```python
from build123d import *

# Parameters (mm, degrees)
SKETCH1_R           = 6.35
BOSS_EXTRUDE1_DEPTH = 38.1
SKETCH2_R           = 9.525
BOSS_EXTRUDE2_DEPTH = 12.7
CUT_EXTRUDE1_DEPTH  = 6.223


with BuildPart() as part:
    # Sketch1 → Boss-Extrude1 (new body)
    with BuildSketch(Plane(origin=(0, 0, 0), x_dir=(0, 0, -1), z_dir=(1, 0, 0))):
        Circle(SKETCH1_R)
    extrude(amount=-BOSS_EXTRUDE1_DEPTH)

    # Sketch2 → Boss-Extrude2 (add)
    with BuildSketch(Plane(origin=(0, 0, 0), x_dir=(0, 0, -1), z_dir=(1, 0, 0))):
        Circle(SKETCH2_R)
    extrude(amount=BOSS_EXTRUDE2_DEPTH)

    # Sketch3 → Cut-Extrude1 (cut)
    with BuildSketch(Plane(origin=(12.7, 0, 0), x_dir=(0, 0, -1), z_dir=(1, 0, 0))):
        Polygon((2.749630657, 4.7625), (-2.749630657, 4.7625), (-5.499261314, 0), (-2.749630657, -4.7625), (2.749630657, -4.7625), (5.499261314, 0), align=None)
    extrude(amount=-CUT_EXTRUDE1_DEPTH, mode=Mode.SUBTRACT)


solid = part.part
```
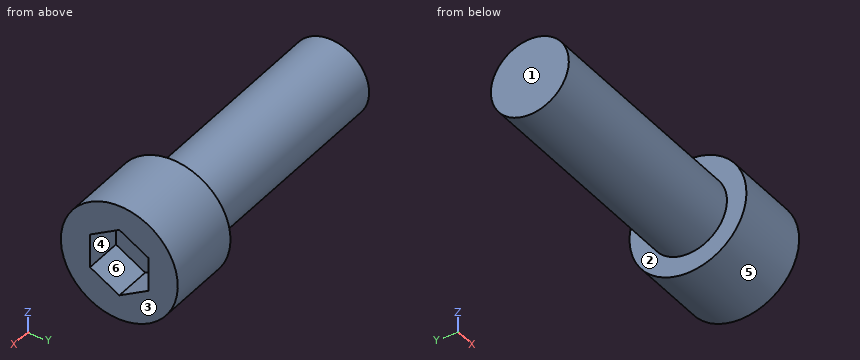
Design review of the part built by this model. Coordinates are the model's own, in mm. Face numbers are marked on the shaded views. A direction names the side the tool comes from. Give positions to 0.01 mm unless a question says otherwise; leave off trailing zeros. Loops run counter-clockwise (first coordinate to the right, second up) from the corner with the lowest first, then second, coordinate; pieces in that order, holes last. Notation, with made-up numbers: (53, 21.25) -> (105, 21.25) arc R18 cw to (105, 36.25) -> close; hole circle Ø11 at (78.25, -21). An arc over 180 degrees is marked (long way). One line per item, written item: value.
Q1. Draft analysis for pull direction Y (two halves, no side actions). For the marked faces 3, 4, 5 and 6, state which applies: pulls with the +Y half, pulls with the -Y half, needs draft (parallel to the pull), parting line crosses it, or undercut.
Numbers:
face 3: needs draft
face 4: undercut
face 5: parting line crosses it
face 6: undercut
Q2. We need section B-B on y = 1.5. Give the boundary of the cut face in (x, z), and give its area (3 significant figures).
Numbers:
outline: (-38.1, -6.17) -> (0, -6.17) -> (0, -9.41) -> (12.7, -9.41) -> (12.7, -4.63) -> (6.48, -4.63) -> (6.48, 4.63) -> (12.7, 4.63) -> (12.7, 9.41) -> (0, 9.41) -> (0, 6.17) -> (-38.1, 6.17) -> close
area: 651 mm^2
Q3. For pin 1 Ø8 at (y, z) = (-7, -0.5) entering from -X; pin 2 Ø5 at (x, z) = (3.5, 4.5) entering from -Y; pin 3 Ø1.5 at (x, y) = (-31, -5.5) entering from +Z; pin 4 Ø4 at (x, z) = (-7, 6) entering from +Y, all flat-tipped, find the tip position at first contact; note any pin that passes through.
Numbers:
pin 1: stops at x = -38.1
pin 2: stops at y = -9.31
pin 3: stops at z = 4.21
pin 4: stops at y = 4.93
Q4. We need section D-D on y = 7.75. Give the boundary of the cut face in (x, z).
Numbers:
outline: (0, -5.54) -> (12.7, -5.54) -> (12.7, 5.54) -> (0, 5.54) -> close
Q5. We need section C-C on x = -8. Give the boundary of the cut face in (y, z).
Numbers:
outline: circle Ø12.7 at (0, 0)
Q6. For L1, parallel to X at y = 4.25, z = 4.75; L2, parallel to Y at x = 9, z = -1.25; L3, parallel to X at y = 0.75, z = 2.25, list the stretches that pass through material, from the lowest coordinate up.
Numbers:
L1: x = 0 to 12.7
L2: y = -9.44 to -4.76, 4.76 to 9.44
L3: x = -38.1 to 6.48
Q7. Machinability: for the marked faces 1 and 2, which of the approach directions +Z, -Z, +X, -X, +Y, -Y give a long, thin tool a straight path to every point of the face, cutting with its end or side? Answer none if there is none.
Numbers:
face 1: +Z, -Z, -X, +Y, -Y
face 2: -X
